```python
from build123d import *

# Parameters (mm, degrees)
F2_DEPTH     = 5
F3_DEPTH     = 3.5
F4_T1_DEPTH  = 14.2822071908
F4_T3_DEPTH  = 11.1004623397
F4_T5_DEPTH  = 14.2822071908
F4_T7_DEPTH  = 11.1004623397
F4_T13_DEPTH = 11.1004623397
F4_T18_DEPTH = 14.2822071908
F4_T26_DEPTH = 14.2822071908
F4_T31_DEPTH = 11.1004623397
F4_T39_DEPTH = 14.2822071908
F4_T44_DEPTH = 11.1004623397
F4_T52_DEPTH = 11.1004623397
F4_T57_DEPTH = 14.2822071908


# Not quite as in the source:
# - a fillet or chamfer that OpenCascade refuses, or shapes differently, is made with other operations: its cross-section is extruded or revolved along the edge and cut away or added


with BuildPart() as f2:
    # F1 (on Top) → F2 (new body)
    with BuildSketch(Plane.XY):
        Polygon((-5.3529168636, -11.2), (5.3529168636, -11.2), (5.3529168636, -5), (15, -5), (15, 5), (5.3529168636, 5), (5.3529168636, 11.2), (-5.3529168636, 11.2), (-5.3529168636, 5), (-15, 5), (-15, -5), (-5.3529168636, -5), align=None)
    extrude(amount=F2_DEPTH)

    # F0 (on Top) → F3 (cut)
    with BuildSketch(Plane.XY):
        Polygon((-3.75, -11.2), (3.75, -11.2), (3.75, -3.75), (15, -3.75), (15, 3.75), (3.75, 3.75), (3.75, 11.2), (-3.75, 11.2), (-3.75, 3.75), (-15, 3.75), (-15, -3.75), (-3.75, -3.75), align=None)
    extrude(amount=F3_DEPTH, mode=Mode.SUBTRACT)

    # F4: fillet of radius 2 on 8 edges, made by hand

    # F4_s2 → F4_t1 (cut)
    with BuildSketch(Plane.YZ.offset(5.3529168636)):
        with BuildLine():
            ThreePointArc((5, 1.8540496218), (4.6583123952, 0.736015633), (3.75, 0))
            Line((3.75, 0), (5, 0))
            Line((5, 0), (5, 1.8540496218))
        make_face()
        with BuildLine():
            ThreePointArc((-5, 1.8540496218), (-4.6583123952, 0.736015633), (-3.75, 0))
            Line((-3.75, 0), (-5, 0))
            Line((-5, 0), (-5, 1.8540496218))
        make_face()
    extrude(amount=F4_T1_DEPTH, mode=Mode.SUBTRACT)

    # F4_s4 → F4_t3 (cut)
    with BuildSketch(Plane.XZ.offset(-16.1004623397)):
        with BuildLine():
            ThreePointArc((-3.75, 0), (-4.9011685022, 0.6941214052), (-5.3529168636, 1.9601849359))
            Line((-5.3529168636, 1.9601849359), (-5.3529168636, 0))
            Line((-5.3529168636, 0), (-3.75, 0))
        make_face()
        with BuildLine():
            ThreePointArc((5.3529168636, 1.9601849359), (4.9011685022, 0.6941214052), (3.75, 0))
            Line((3.75, 0), (5.3529168636, 0))
            Line((5.3529168636, 0), (5.3529168636, 1.9601849359))
        make_face()
    extrude(amount=F4_T3_DEPTH, mode=Mode.SUBTRACT)

    # F4_s6 → F4_t5 (cut)
    with BuildSketch(Plane.YZ.offset(-19.6351240544)):
        with BuildLine():
            ThreePointArc((3.75, 0), (4.6583123952, 0.736015633), (5, 1.8540496218))
            Line((5, 1.8540496218), (5, 0))
            Line((5, 0), (3.75, 0))
        make_face()
        with BuildLine():
            ThreePointArc((-5, 1.8540496218), (-4.6583123952, 0.736015633), (-3.75, 0))
            Line((-3.75, 0), (-5, 0))
            Line((-5, 0), (-5, 1.8540496218))
        make_face()
    extrude(amount=F4_T5_DEPTH, mode=Mode.SUBTRACT)

    # F4_s8 → F4_t7 (cut)
    with BuildSketch(Plane.XZ.offset(5)):
        with BuildLine():
            ThreePointArc((-5.3529168636, 1.9601849359), (-4.9011685022, 0.6941214052), (-3.75, 0))
            Line((-3.75, 0), (-5.3529168636, 0))
            Line((-5.3529168636, 0), (-5.3529168636, 1.9601849359))
        make_face()
        with BuildLine():
            ThreePointArc((5.3529168636, 1.9601849359), (4.9011685022, 0.6941214052), (3.75, 0))
            Line((3.75, 0), (5.3529168636, 0))
            Line((5.3529168636, 0), (5.3529168636, 1.9601849359))
        make_face()
    extrude(amount=F4_T7_DEPTH, mode=Mode.SUBTRACT)


with BuildPart() as f4_tool11:
    # F4_s12 → F4_t13 (new body)
    with BuildSketch(Plane.XZ.offset(-0.0995376603)):
        with BuildLine():
            ThreePointArc((5.3529168636, 1.9601849359), (4.9011685022, 0.6941214052), (3.75, 0))
            Line((3.75, 0), (5.3529168636, 0))
            Line((5.3529168636, 0), (5.3529168636, 1.9601849359))
        make_face()
    extrude(amount=-F4_T13_DEPTH)

    split(bisect_by=Plane.XZ.offset(-5), keep=Keep.TOP)

    split(bisect_by=Plane.XZ.offset(-3.75), keep=Keep.BOTTOM)


with BuildPart() as f4_tool16:
    # F4_s17 → F4_t18 (new body)
    with BuildSketch(Plane.YZ.offset(15)):
        with BuildLine():
            ThreePointArc((5, 1.8540496218), (4.6583123952, 0.736015633), (3.75, 0))
            Line((3.75, 0), (5, 0))
            Line((5, 0), (5, 1.8540496218))
        make_face()
    extrude(amount=-F4_T18_DEPTH)

    split(bisect_by=Plane.YZ.offset(5.3529168636), keep=Keep.BOTTOM)

    split(bisect_by=Plane.YZ.offset(3.75), keep=Keep.TOP)


with BuildPart() as f4_tool11_1:
    add(f4_tool11.part)

    # F4_t21: intersect F4_tool16
    add(f4_tool16.part, mode=Mode.INTERSECT)


with BuildPart() as f2_1:
    add(f2.part)

    # F4_t9: cut F4_tool11
    add(f4_tool11_1.part, mode=Mode.SUBTRACT)


with BuildPart() as f4_tool24:
    # F4_s25 → F4_t26 (new body)
    with BuildSketch(Plane.YZ.offset(-0.7177928092)):
        with BuildLine():
            ThreePointArc((3.75, 0), (4.6583123952, 0.736015633), (5, 1.8540496218))
            Line((5, 1.8540496218), (5, 0))
            Line((5, 0), (3.75, 0))
        make_face()
    extrude(amount=-F4_T26_DEPTH)

    split(bisect_by=Plane.YZ.offset(-3.75), keep=Keep.BOTTOM)

    split(bisect_by=Plane.YZ.offset(-5.3529168636), keep=Keep.TOP)


with BuildPart() as f4_tool29:
    # F4_s30 → F4_t31 (new body)
    with BuildSketch(Plane.XZ.offset(-11.2)):
        with BuildLine():
            ThreePointArc((-3.75, 0), (-4.9011685022, 0.6941214052), (-5.3529168636, 1.9601849359))
            Line((-5.3529168636, 1.9601849359), (-5.3529168636, 0))
            Line((-5.3529168636, 0), (-3.75, 0))
        make_face()
    extrude(amount=F4_T31_DEPTH)

    split(bisect_by=Plane.XZ.offset(-5), keep=Keep.TOP)

    split(bisect_by=Plane.XZ.offset(-3.75), keep=Keep.BOTTOM)


with BuildPart() as f4_tool24_1:
    add(f4_tool24.part)

    # F4_t34: intersect F4_tool29
    add(f4_tool29.part, mode=Mode.INTERSECT)


with BuildPart() as f2_2:
    add(f2_1.part)

    # F4_t22: cut F4_tool24
    add(f4_tool24_1.part, mode=Mode.SUBTRACT)


with BuildPart() as f4_tool37:
    # F4_s38 → F4_t39 (new body)
    with BuildSketch(Plane.YZ.offset(-15)):
        with BuildLine():
            ThreePointArc((-5, 1.8540496218), (-4.6583123952, 0.736015633), (-3.75, 0))
            Line((-3.75, 0), (-5, 0))
            Line((-5, 0), (-5, 1.8540496218))
        make_face()
    extrude(amount=F4_T39_DEPTH)

    split(bisect_by=Plane.YZ.offset(-5.3529168636), keep=Keep.TOP)

    split(bisect_by=Plane.YZ.offset(-3.75), keep=Keep.BOTTOM)


with BuildPart() as f4_tool42:
    # F4_s43 → F4_t44 (new body)
    with BuildSketch(Plane.XZ.offset(0.0995376603)):
        with BuildLine():
            ThreePointArc((-5.3529168636, 1.9601849359), (-4.9011685022, 0.6941214052), (-3.75, 0))
            Line((-3.75, 0), (-5.3529168636, 0))
            Line((-5.3529168636, 0), (-5.3529168636, 1.9601849359))
        make_face()
    extrude(amount=F4_T44_DEPTH)

    split(bisect_by=Plane.XZ.offset(5), keep=Keep.BOTTOM)

    split(bisect_by=Plane.XZ.offset(3.75), keep=Keep.TOP)


with BuildPart() as f4_tool37_1:
    add(f4_tool37.part)

    # F4_t47: intersect F4_tool42
    add(f4_tool42.part, mode=Mode.INTERSECT)


with BuildPart() as f2_3:
    add(f2_2.part)

    # F4_t35: cut F4_tool37
    add(f4_tool37_1.part, mode=Mode.SUBTRACT)


with BuildPart() as f4_tool50:
    # F4_s51 → F4_t52 (new body)
    with BuildSketch(Plane.XZ.offset(11.2)):
        with BuildLine():
            ThreePointArc((5.3529168636, 1.9601849359), (4.9011685022, 0.6941214052), (3.75, 0))
            Line((3.75, 0), (5.3529168636, 0))
            Line((5.3529168636, 0), (5.3529168636, 1.9601849359))
        make_face()
    extrude(amount=-F4_T52_DEPTH)

    split(bisect_by=Plane.XZ.offset(5), keep=Keep.BOTTOM)

    split(bisect_by=Plane.XZ.offset(3.75), keep=Keep.TOP)


with BuildPart() as f4_tool55:
    # F4_s56 → F4_t57 (new body)
    with BuildSketch(Plane.YZ.offset(0.7177928092)):
        with BuildLine():
            ThreePointArc((-5, 1.8540496218), (-4.6583123952, 0.736015633), (-3.75, 0))
            Line((-3.75, 0), (-5, 0))
            Line((-5, 0), (-5, 1.8540496218))
        make_face()
    extrude(amount=F4_T57_DEPTH)

    split(bisect_by=Plane.YZ.offset(5.3529168636), keep=Keep.BOTTOM)

    split(bisect_by=Plane.YZ.offset(3.75), keep=Keep.TOP)


with BuildPart() as f4_tool50_1:
    add(f4_tool50.part)

    # F4_t60: intersect F4_tool55
    add(f4_tool55.part, mode=Mode.INTERSECT)


with BuildPart() as f2_4:
    add(f2_3.part)

    # F4_t48: cut F4_tool50
    add(f4_tool50_1.part, mode=Mode.SUBTRACT)


solid = f2_4.part
```
Can you work these out from the model? Positions are in its coordinate system, mm. A direction names the side the tool comes from. Coordinates: 2 decimals unless noted, no trailing zeros. Loops run counter-clockwise (first coordinate to the right, second up) from the corner with the lowest first, then second, coordinate; pieces in that order, holes last.
1) I need wall thicknesses on probe 1 along X at (y, z) = (-4.5, 1.1); probe 2 along Y at (x, z) = (6.5, 2.8); probe 3 along X at (y, z) = (9.5, 3.05). Which ranges of each line are inside material? Lowest first, please.
2) Imagine slicing it at B-B on x = -11. List the corners of the cut face in (y, z) for me, plus the area to 3 significant figures.
3) Imagine slicing it at C-C on y = -6.75. List the corners of the cut face in (x, z) for me, plus the area to 3 significant figures.
4) Imagine slicing it at D-D on z = 1.45. List the corners of the cut face in (x, y) for me, plus the area to 3 significant figures.
5) For pin 1 (1 mm diameter, centred on y = -9, z = 1.5, fed in from -X); pin 2 (6 mm diameter, centred on x = -7, y = 4.5, fed in from -Z); pin 3 (1.5 mm diameter, centred on x = -11, z = 2, fed in from -Y), each with a flat end and sliding along its axis, tell me the tip position at first contact or that it passes through.
6) Which directions (+Z, -Z, +X, -X, +Y, -Y) give clear straight access to the entire face, cutting with the end or side of a thin tool? Please do faces 4 (the flat face through (-9, 3.75, 2)), 5 (the flat face through (-10, -5, 3)), 6 (the flat face through (5.353, -8, 3)), 7 (the flat face through (3.75, -8, 2)), 8 (the flat face through (-10, 5, 3)).
7) Imagine slicing it at A-A on z = 3. List the corners of the cut face in (x, y) for me.
8) Thinking about a two-plate mould opening in X: for faces 1 (the flat face through (-3.75, 8, 2)), 2 (the flat face through (-9, -3.75, 2)), 3 (the flat face through (15, 0, 4)), which applies, pulls with the +X half, pulls with the -X half, needs draft (parallel to the pull), parting line crosses it, or undercut?
Completed:
1. probe 1: x = -15 to -3.75, 3.75 to 15
1. probe 2: y = -5 to -3.75, 3.75 to 5
1. probe 3: x = -5.35 to -3.75, 3.75 to 5.35
2. outline: (-5, 1.85) arc R2 ccw to (-3.75, 0) - (-3.75, 3.5) - (3.75, 3.5) - (3.75, 0) arc R2 ccw to (5, 1.85) - (5, 5) - (-5, 5) - close
2. area: 22.5 mm2
3. outline: (-5.35, 1.96) arc R2 ccw to (-3.75, 0) - (-3.75, 3.5) - (3.75, 3.5) - (3.75, 0) arc R2 ccw to (5.35, 1.96) - (5.35, 5) - (-5.35, 5) - close
3. area: 25.7 mm2
4. outline: (-15, -4.96) - (-5.29, -4.96) - (-5.29, -11.2) - (-3.75, -11.2) - (-3.75, -3.75) - (-15, -3.75) - close; (-15, 3.75) - (-3.75, 3.75) - (-3.75, 11.2) - (-5.29, 11.2) - (-5.29, 4.96) - (-15, 4.96) - close; (3.75, -11.2) - (5.29, -11.2) - (5.29, -4.96) - (15, -4.96) - (15, -3.75) - (3.75, -3.75) - close; (3.75, 3.75) - (15, 3.75) - (15, 4.96) - (5.29, 4.96) - (5.29, 11.2) - (3.75, 11.2) - close
4. area: 92.8 mm2
5. pin 1: stops at x = -5.35
5. pin 2: stops at z = 0
5. pin 3: stops at y = -5
6. face 4: -Z, +X, -X
6. face 5: +Z, -Z, -X, -Y
6. face 6: +Z, -Z, +X, -Y
6. face 7: -Z, +Y, -Y
6. face 8: +Z, -Z, -X, +Y
7. outline: (-15, -5) - (-5.35, -5) - (-5.35, -11.2) - (-3.75, -11.2) - (-3.75, -3.75) - (-15, -3.75) - close; (-15, 3.75) - (-3.75, 3.75) - (-3.75, 11.2) - (-5.35, 11.2) - (-5.35, 5) - (-15, 5) - close; (3.75, -11.2) - (5.35, -11.2) - (5.35, -5) - (15, -5) - (15, -3.75) - (3.75, -3.75) - close; (3.75, 3.75) - (15, 3.75) - (15, 5) - (5.35, 5) - (5.35, 11.2) - (3.75, 11.2) - close
8. face 1: undercut
8. face 2: needs draft
8. face 3: pulls with the +X half
